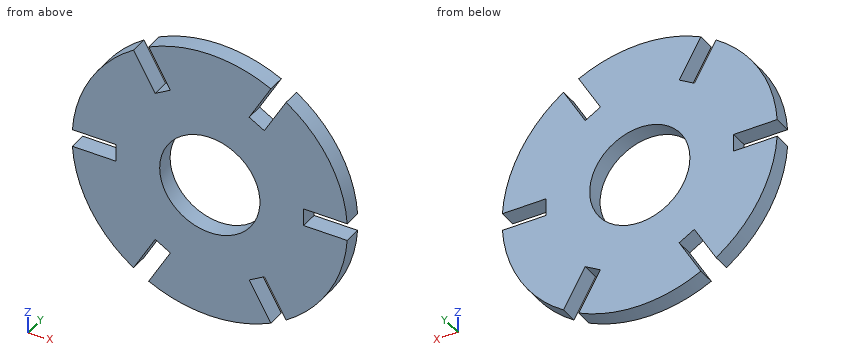
Autodesk Inventor part; units mm, degrees
ref_plane "YZ Plane" through (0, 0, 0) normal (1, 0, 0) x (0, 1, 0)
ref_plane "XZ Plane" through (0, 0, 0) normal (0, 1, 0) x (-1, 0, 0)
ref_plane "XY Plane" through (0, 0, 0) normal (0, 0, 1) x (1, 0, 0)
sketch "Sketch1" plane through (0, 0, 0) normal (0, 1, 0) x (-1, 0, 0)
  circle A0 centre (0, 0) radius 15.725
  circle A1 centre (0, 0) radius 5.725
  dimension "d0" = 31.45
  dimension "d1" = 11.45
extrude "Extrusion1" add sketch "Sketch1" along normal blind 2
sketch "Sketch2" plane through (0, 2, 0) normal (0, 1, 0) x (1, 0, 0)
  line L0 (-20.725, -1) -> (-10.725, -1)
  line L1 (-10.725, -1) -> (-10.725, 1)
  line L2 (-10.725, 1) -> (-20.725, 1)
  line L3 (-20.725, 1) -> (-20.725, -1)
  point P0 (0, 0)
  dimension "d4" = 1
  dimension "d5" = 2
  dimension "d6" = 10
  dimension "d7" = 10.725
extrude "Extrusion2" cut sketch "Sketch2" against normal blind 2
pattern_circular "Circular Pattern1" count 6 over 360 about axis through (0, -10, 0) along (0, 1, 0) of "Extrusion2"
properties part number "Ring_n8"
Input: part model. Units: mm. Frame: model coordinates. Give positions to 0.01 mm unless a question says otherwise; leave off trailing zeros. Loops run counter-clockwise (first coordinate to the right, second up) from the corner with the lowest first, then second, coordinate; pieces in that order, holes last.
1) Section query A-A on z = 0. Return the cut outline in (x, y) (3 decimals).
A:
outline: (-10.725, 0) - (-5.725, 0) - (-5.725, 2) - (-10.725, 2) - close; (5.725, 0) - (10.725, 0) - (10.725, 2) - (5.725, 2) - close
2) Contact query for flat-ended pins moving along their axis: pin 1 (0.6 mm diameter, centred on y = 1, z = -0.5, fed in from +X) (3 decimals); pin 2 (1 mm diameter, centred on y = 2, z = 4, fed in from -X); pin 3 (1 mm diameter, centred on y = 0.5, z = 0, fed in from -X) (3 decimals). Output: stop coordinate, or through.
A:
pin 1: stops at x = 10.725
pin 2: stops at x = -15.33
pin 3: stops at x = -10.725
3) Section query B-B on x = 0. Return the cut outline in (y, z) (3 decimals).
A:
outline: (0, -15.725) - (2, -15.725) - (2, -5.725) - (0, -5.725) - close; (0, 5.725) - (2, 5.725) - (2, 15.725) - (0, 15.725) - close
4) Line query: L1, parallel to Z at x = 0, y = 1.55 (3 decimals); L2, parallel to X at y = 1.15, z = 13; L3, parallel to Z at x = 6, y = 1.8. Output: solid intervals per line, ascending.
A:
L1: z = -15.725 to -5.725, 5.725 to 15.725
L2: x = -8.85 to -8.66, -6.35 to 6.35, 8.66 to 8.85
L3: z = -14.54 to -12.39, -8.92 to 8.92, 12.39 to 14.54
5) Section query C-C on x = 5. Return the cut outline in (y, z).
A:
outline: (0, -14.91) - (2, -14.91) - (2, -10.66) - (0, -10.66) - close; (0, -9.5) - (2, -9.5) - (2, -2.79) - (0, -2.79) - close; (0, 2.79) - (2, 2.79) - (2, 9.5) - (0, 9.5) - close; (0, 10.66) - (2, 10.66) - (2, 14.91) - (0, 14.91) - close
